Read the model definition and answer for the solid it produces. Units are mm, in the model's axes. Face numbers are marked on the shaded views. A direction names the side the tool comes from. Give positions to 0.01 mm unless a question says otherwise; leave off trailing zeros. Order: outer loops, then holes, each group sorted by start corner. A loop starts at its lowest first (then second) coordinate and runs counter-clockwise, first axis right, second up.
```python
from build123d import *

# Parameters (mm, degrees)
SKETCH1_R             = 2.55
BOSS_EXTRUDE1_DEPTH   = 1.57
SKETCH2_W             = 1.57
SKETCH2_H             = 3.18
BOSS_EXTRUDE2_DEPTH   = 4.75
SKETCH3_W             = 3.96
SKETCH3_H             = 1.57
BOSS_EXTRUDE3_DEPTH   = 2.39
FILLET1_R             = 1.57
CHAMFER1_SIZE         = 3
CHAMFER1_SIZE2        = 0.262465991
CHAMFER1_PART_2_SIZE  = 3
CHAMFER1_PART_2_SIZE2 = 0.262465991
CHAMFER1_PART_3_SIZE  = 3
CHAMFER1_PART_3_SIZE2 = 0.262465991
CHAMFER1_PART_4_SIZE  = 3
CHAMFER1_PART_4_SIZE2 = 0.262465991


with BuildPart() as part:
    # Sketch1 → Boss-Extrude1 (new body)
    with BuildSketch(Plane(origin=(0, 0, 0), x_dir=(1, 0, 0), z_dir=(0, 1, 0))):
        with BuildLine():
            Line((-4.76, 2.853927119), (-4.76, 1.59))
            Line((-4.76, 1.59), (-6.74, 1.59))
            Line((-6.74, 1.59), (-6.74, -1.59))
            Line((-6.74, -1.59), (-4.76, -1.59))
            Line((-4.76, -1.59), (-4.76, -2.853927119))
            ThreePointArc((-4.76, -2.853927119), (0, -5.55), (4.76, -2.853927119))
            Line((4.76, -2.853927119), (4.76, -1.59))
            Line((4.76, -1.59), (6.74, -1.59))
            Line((6.74, -1.59), (6.74, 1.59))
            Line((6.74, 1.59), (4.76, 1.59))
            Line((4.76, 1.59), (4.76, 2.853927119))
            ThreePointArc((4.76, 2.853927119), (3.565828986, 4.252924128), (1.98, 5.184795078))
            Line((1.98, 5.184795078), (1.98, 7.92))
            Line((1.98, 7.92), (-1.98, 7.92))
            Line((-1.98, 7.92), (-1.98, 5.184795078))
            ThreePointArc((-1.98, 5.184795078), (-3.565828986, 4.252924128), (-4.76, 2.853927119))
        make_face()
        Circle(SKETCH1_R, mode=Mode.SUBTRACT)
    extrude(amount=BOSS_EXTRUDE1_DEPTH)

    # Sketch2 → Boss-Extrude2 (add)
    with BuildSketch(Plane.XZ):
        with Locations((-5.955, 0)):
            Rectangle(SKETCH2_W, SKETCH2_H)
        with Locations((5.955, 0)):
            Rectangle(SKETCH2_W, SKETCH2_H)
    extrude(amount=BOSS_EXTRUDE2_DEPTH)

    # Sketch3 → Boss-Extrude3 (add)
    with BuildSketch(Plane(origin=(0, 1.57, 0), x_dir=(1, 0, 0), z_dir=(0, 1, 0))):
        with Locations((0, 7.135)):
            Rectangle(SKETCH3_W, SKETCH3_H)
    extrude(amount=BOSS_EXTRUDE3_DEPTH)

    # Fillet1
    fillet1_edges = [part.edges().sort_by_distance(p)[0] for p in [
        (0, 0, -7.92),
        (6.74, 1.57, 0),
        (-6.74, 1.57, 0),
    ]]
    fillet(fillet1_edges, radius=FILLET1_R)

    # Chamfer1
    chamfer1_edges = [part.edges().sort_by_distance(p)[0] for p in [
        (5.955, -4.75, -1.59),
    ]]
    chamfer1_side = [part.faces().sort_by_distance(p)[0] for p in [
        (5.8686205, -1.585741835, -1.59),
    ]]
    chamfer(chamfer1_edges, length=CHAMFER1_SIZE, length2=CHAMFER1_SIZE2, reference=chamfer1_side[0])

    # Chamfer1 part 2
    chamfer1_part_2_edges = [part.edges().sort_by_distance(p)[0] for p in [
        (5.955, -4.75, 1.59),
    ]]
    chamfer1_part_2_side = [part.faces().sort_by_distance(p)[0] for p in [
        (5.8686205, -1.585741835, 1.59),
    ]]
    chamfer(chamfer1_part_2_edges, length=CHAMFER1_PART_2_SIZE, length2=CHAMFER1_PART_2_SIZE2, reference=chamfer1_part_2_side[0])

    # Chamfer1 part 3
    chamfer1_part_3_edges = [part.edges().sort_by_distance(p)[0] for p in [
        (-5.955, -4.75, -1.59),
    ]]
    chamfer1_part_3_side = [part.faces().sort_by_distance(p)[0] for p in [
        (-5.8686205, -1.585741835, -1.59),
    ]]
    chamfer(chamfer1_part_3_edges, length=CHAMFER1_PART_3_SIZE, length2=CHAMFER1_PART_3_SIZE2, reference=chamfer1_part_3_side[0])

    # Chamfer1 part 4
    chamfer1_part_4_edges = [part.edges().sort_by_distance(p)[0] for p in [
        (-5.955, -4.75, 1.59),
    ]]
    chamfer1_part_4_side = [part.faces().sort_by_distance(p)[0] for p in [
        (-5.8686205, -1.585741835, 1.59),
    ]]
    chamfer(chamfer1_part_4_edges, length=CHAMFER1_PART_4_SIZE, length2=CHAMFER1_PART_4_SIZE2, reference=chamfer1_part_4_side[0])


solid = part.part
```
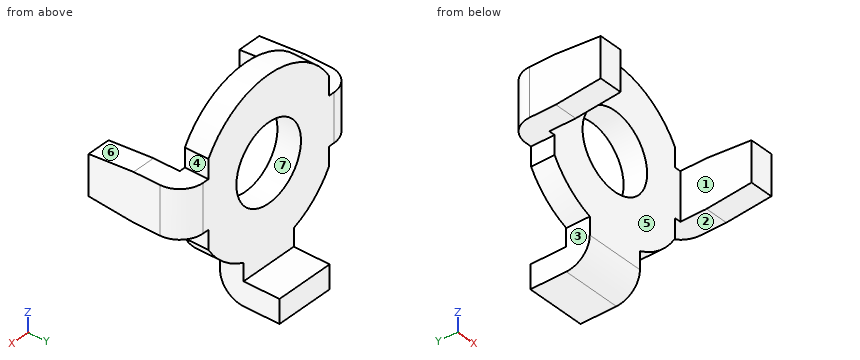
1) The part is cut by section B-B on x = 0. Determine the outline of the cut face in (y, z), and give its area (3 significant figures).
Final values:
outline: (0, -6.35) arc R1.57 ccw to (1.57, -7.92) - (3.96, -7.92) - (3.96, -6.35) - (1.57, -6.35) - (1.57, -2.55) - (0, -2.55) - close; (0, 2.55) - (1.57, 2.55) - (1.57, 5.55) - (0, 5.55) - close
area: 16.4 mm2
2) Given pin 1 (1 mm diameter, centred on y = 1, z = 3, fed in from +X); pin 2 (0.6 mm diameter, centred on x = -6, y = -1, fed in from +Z); pin 3 (5 mm diameter, centred on y = 2.5, z = -0.5, fed in from -X); pin 4 (4 mm diameter, centred on x = 0, z = 0, fed in from +Y), each flat-ended and moving along its own axis, determine where each tip first touches the part or whether it passes through.
Final values:
pin 1: stops at x = 4.76
pin 2: stops at z = 1.59
pin 3: stops at x = -6.74
pin 4: passes through
3) The part is cut by section C-C on z = 2.25. Determine the outline of the cut face in (x, y), and give its area (3 significant figures).
Final values:
outline: (-4.76, 0) - (-1.2, 0) - (-1.2, 1.57) - (-4.76, 1.57) - close; (1.2, 0) - (4.76, 0) - (4.76, 1.57) - (1.2, 1.57) - close
area: 11.2 mm2
4) A tool of negligible diameter and unlimited length cuts with its end or side. For the marked faces 1, 2 and 3, from which of +Z, -Z, +X, -X, +Y, -Y can it reach the whole face along a straight path? Write none if from no direction.
Final values:
face 1: +Z, -Z, -Y
face 2: -Z, +X, +Y, -Y
face 3: -Z, -X, +Y, -Y
5) Consider L1, parallel to X at y = -1.5, z = -0.75; L2, parallel to Y at x = -3.5, z = -1.25; L3, parallel to X at y = 0.3, z = 0. Determine where each line is inside the solid, lowest interval first.
Final values:
L1: x = -6.74 to -5.17, 5.17 to 6.74
L2: y = 0 to 1.57
L3: x = -6.71 to -2.55, 2.55 to 6.71
6) The part is cut by section A-A on y = -3. Determine the outline of the cut face in (x, z), and give its area (3 significant figures).
Final values:
outline: (-6.74, -1.48) - (-5.17, -1.48) - (-5.17, 1.48) - (-6.74, 1.48) - close; (5.17, -1.48) - (6.74, -1.48) - (6.74, 1.48) - (5.17, 1.48) - close
area: 9.30 mm2
7) The part is cut by section D-D on z = -0.5. Determine the outline of the cut face in (x, y).
Final values:
outline: (-6.74, -4.75) - (-5.17, -4.75) - (-5.17, 0) - (-2.5, 0) - (-2.5, 1.57) - (-5.17, 1.57) arc R1.57 ccw to (-6.74, 0) - close; (2.5, 0) - (5.17, 0) - (5.17, -4.75) - (6.74, -4.75) - (6.74, 0) arc R1.57 ccw to (5.17, 1.57) - (2.5, 1.57) - close
8) For a pull along X with two mould halves and no side action, classify the marked faces 4, 5, 6 and 7 as released by +X, released by -X, zero draft, split by the parting line, or undercut.
Final values:
face 4: released by +X
face 5: undercut
face 6: zero draft
face 7: undercut
